Autodesk Inventor part; units mm, degrees
ref_plane "YZ Plane" through (0, 0, 0) normal (1, 0, 0) x (0, 1, 0)
ref_plane "XZ Plane" through (0, 0, 0) normal (0, 1, 0) x (-1, 0, 0)
ref_plane "XY Plane" through (0, 0, 0) normal (0, 0, 1) x (1, 0, 0)
sketch "Sketch1" plane through (0, 0, 0) normal (0, 0, 1) x (1, 0, 0)
  line L0 (57.15, -25.4) -> (-57.15, -25.4)
  line L1 (-57.15, -25.4) -> (-57.15, 25.4)
  line L2 (-57.15, 25.4) -> (57.15, 25.4)
  line L3 (57.15, 25.4) -> (57.15, -25.4)
  line L4 (57.15, -25.4) -> (-57.15, 25.4) construction
  line L5 (-57.15, -25.4) -> (57.15, 25.4) construction
  point P0 (0, 0)
  point P1 (0, 0)
  point P2 (0, 0)
  dimension "d0" = 114.3
  dimension "d1" = 50.8
extrude "Extrusion1" add sketch "Sketch1" along normal blind 19.05
sketch "Sketch2" plane through (0, 0, 19.05) normal (0, 0, 1) x (1, 0, 0)
  circle A0 centre (0, -26.67) radius 32.258
  line L0 (-57.15, -25.4) -> (57.15, -25.4)
  line L1 (-57.15, 25.4) -> (-57.15, -25.4)
  point P0 (0, 0)
  dimension "d4" = 64.516
  dimension "d6" = 1.27
  dimension "d48" = 57.15
extrude "Extrusion2" cut sketch "Sketch2" against normal through all
sketch "Sketch4" plane through (-57.15, 25.4, 0) normal (0, 1, 0) x (1, 0, 0)
  circle A0 centre (15.875, -9.525) radius 3.3734
  circle A1 centre (98.425, -9.525) radius 3.3734
  line L0 (114.3, 0) -> (0, 0)
  line L1 (57.15, -22.86) -> (57.15, 3.81)
  dimension "d27" = 6.7469
  dimension "d28" = 9.525
  dimension "d49" = 41.275
  dimension "d50" = 41.275
extrude "Extrusion4" cut sketch "Sketch4" against normal through all
sketch "Sketch5" plane through (-57.15, -25.4, 0) normal (0, -1, 0) x (1, 0, 0)
  circle A0 centre (6.35, 9.525) radius 2.0193
  circle A1 centre (107.95, 9.525) radius 2.0193
  line L0 (0, 0) -> (24.917, 0)
  line L1 (57.15, 22.86) -> (57.15, -3.81)
  dimension "d33" = 9.525
  dimension "d34" = 4.0386
  dimension "d51" = 50.8
  dimension "d52" = 50.8
extrude "Extrusion5" cut sketch "Sketch5" against normal through all
sketch "Sketch6" plane through (0, 0, 19.05) normal (0, 0, 1) x (1, 0, 0)
  circle A0 centre (-26.9408, 0.2708) radius 2.5797
  arc A1 (32.233, -25.4) -> (-32.233, -25.4) centre (0, -26.67) ccw
  circle A2 centre (0, 11.43) radius 2.5797
  circle A3 centre (26.9408, 0.2708) radius 2.5797
  line L0 (0, -26.67) -> (0, -14.487)
  dimension "d39" = 38.1
  dimension "d40" = 5.1594
  dimension "d44" = 90
  dimension "d53" = 45
extrude "Extrusion6" cut sketch "Sketch6" against normal through all
equation "\"d50\" = d49"
equation "\"d52\" = d51"
properties part number "ShooterSeperableClampA"
Input: part model. Units: mm. Frame: model coordinates. Give positions to 0.01 mm unless a question says otherwise; leave off trailing zeros. Order: outer loops, then holes, each group sorted by start corner. A loop starts at its lowest first (then second) coordinate and runs counter-clockwise, first axis right, second up. Notation, with made-up numbers: (58, 32) - (102, 32) arc R15 cw to (102, 60) - close; hole circle Ø2 at (12, 23.5). An arc over 180 degrees is marked (long way). Use a Markdown table: item, result.
(1) Draft query along X for faces 1 (the flat face through (57.15, 0, 9)), 2 (the cylindrical face through (52.726, -0.356, 10.132)), 3 (the flat face through (-1, 6, 0)). Return one class per face: released by +X, released by -X, zero draft, split by the parting line, or undercut.
Computed values:
| item | result |
|---|---|
| face 1 | released by +X |
| face 2 | undercut |
| face 3 | zero draft |
(2) Line query: line 1 (X direction, y = -8, z = 12); line 2 (X direction, y = -10, z = 9.75); line 3 (X direction, y = -7, z = 10.75). Output: solid intervals per line, ascending. Write a range as from..to.
Computed values:
| item | result |
|---|---|
| line 1 | x = -57.15..-43.57, -38.98..-26.31, 26.31..38.98, 43.57..57.15 |
| line 2 | x = -57.15..-52.81, -48.79..-44.64, -37.91..-27.62, 27.62..37.91, 44.64..48.79, 52.81..57.15 |
| line 3 | x = -57.15..-52.41, -49.19..-44.42, -38.13..-25.57, 25.57..38.13, 44.42..49.19, 52.41..57.15 |
(3) Section query D-D (z = 15.25). Output: boundary loops of the cut face in (x, y).
Computed values:
| item | result |
|---|---|
| outline | (-57.15, -25.4) - (-32.23, -25.4) arc R32.26 cw to (32.23, -25.4) - (57.15, -25.4) - (57.15, 25.4) - (-57.15, 25.4) - close; hole circle Ø5.16 at (-26.94, 0.27); hole circle Ø5.16 at (0, 11.43); hole circle Ø5.16 at (26.94, 0.27) |
(4) Pin query (flat end, axial travel): pin 1 (8.5 mm diameter, centred on x = 26.94, y = 0.27, fed in from +Z). Return the tip coordinate at first contact, or that it passes through.
Computed values:
| item | result |
|---|---|
| pin 1 | stops at z = 19.05 |
(5) Section query A-A (y = -21.5). Output: boundary loops of the cut face in (x, z) (3 decimals), then the cut area to 3 significant figures.
Computed values:
| item | result |
|---|---|
| outline | (-57.15, 0) - (-31.841, 0) - (-31.841, 19.05) - (-57.15, 19.05) - close; (31.841, 0) - (57.15, 0) - (57.15, 19.05) - (31.841, 19.05) - close; hole circle Ø4.039 at (-50.8, 9.525); hole circle Ø6.747 at (-41.275, 9.525); hole circle Ø6.747 at (41.275, 9.525); hole circle Ø4.039 at (50.8, 9.525) |
| area | 867 mm2 |
(6) Section query B-B (x = 50.8). Output: boundary loops of the cut face in (y, z), then the cut area to 3 significant figures.
Computed values:
| item | result |
|---|---|
| outline | (-25.4, 0) - (25.4, 0) - (25.4, 7.51) - (-25.4, 7.51) - close; (-25.4, 11.54) - (25.4, 11.54) - (25.4, 19.05) - (-25.4, 19.05) - close |
| area | 763 mm2 |
(7) Section query C-C (y = -7). Output: boundary loops of the cut face in (x, z) (3 decimals).
Computed values:
| item | result |
|---|---|
| outline | (-57.15, 0) - (-25.567, 0) - (-25.567, 19.05) - (-57.15, 19.05) - close; (25.567, 0) - (57.15, 0) - (57.15, 19.05) - (25.567, 19.05) - close; hole circle Ø4.039 at (-50.8, 9.525); hole circle Ø6.747 at (-41.275, 9.525); hole circle Ø6.747 at (41.275, 9.525); hole circle Ø4.039 at (50.8, 9.525) |
